Check sheet for the modelled part. Datum: model origin and axes. Units: mm. Face numbers are marked on the shaded views. A direction names the side the tool comes from. Give positions to 0.01 mm unless a question says otherwise; leave off trailing zeros. Write each loop counter-clockwise with the first axis right and the second up, starting at its lowest first coordinate (ties: lowest second). Pieces come first, ordered by that corner, then holes. Notation, with made-up numbers: M 86,16 L 103,16 A33 cw 103,46 Z; hole C 71.5,40 d2. An arc over 180 degrees is marked long. Write each question's results on one line, items separated by ' | '. Start each with the question number.
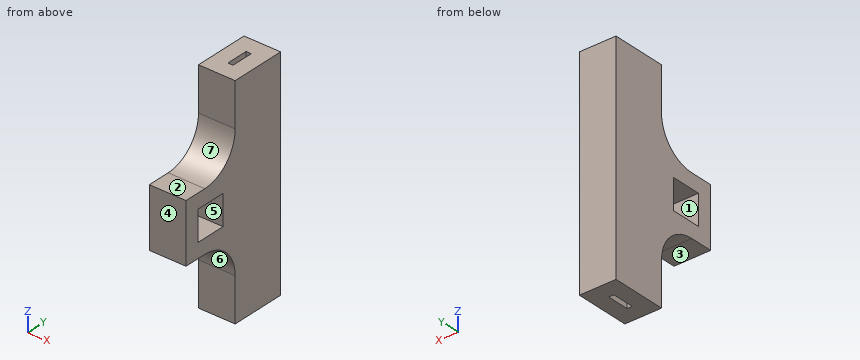
Autodesk Inventor part; units mm, degrees
ref_plane "YZ Plane" through (0, 0, 0) normal (1, 0, 0) x (0, 1, 0)
ref_plane "XZ Plane" through (0, 0, 0) normal (0, 1, 0) x (-1, 0, 0)
ref_plane "XY Plane" through (0, 0, 0) normal (0, 0, 1) x (1, 0, 0)
sketch "Sketch1" plane through (0, 0, 0) normal (1, 0, 0) x (0, 1, 0)
  line L0 (4.05, 4.05) -> (-4.05, 4.05)
  line L1 (-4.05, 4.05) -> (-4.05, -4.05)
  line L2 (-4.05, -4.05) -> (4.05, -4.05)
  line L3 (4.05, -4.05) -> (4.05, 4.05)
  line L4 (11.55, 15) -> (4.05, 15)
  line L5 (4.05, 15) -> (4.05, -15)
  line L6 (4.05, -15) -> (11.55, -15)
  line L7 (11.55, -15) -> (11.55, 15)
  line L8 (4.05, 4.05) -> (-4.05, -4.05) construction
  line L9 (4.05, -4.05) -> (-4.05, 4.05) construction
  line L10 (2.05, 2.05) -> (-2.05, 2.05)
  line L11 (-2.05, 2.05) -> (-2.05, -2.05)
  line L12 (-2.05, -2.05) -> (2.05, -2.05)
  line L13 (2.05, -2.05) -> (2.05, 2.05)
  line L14 (2.05, 2.05) -> (-2.05, -2.05) construction
  line L15 (-2.05, 2.05) -> (2.05, -2.05) construction
  point P0 (4.05, 4.05)
  point P1 (0, 0)
  point P2 (0, 0)
  point P3 (0, 0)
  dimension "d0" = 8.1
  dimension "d3" = 8.1
  dimension "d22" = 10.95
  dimension "d24" = 30
  dimension "d25" = 7.5
  dimension "d55" = 10.95
  dimension "d65" = 4.1
  dimension "d66" = 4.1
extrude "Extrusion1" add sketch "Sketch1" along normal blind 5
sketch "Sketch5" plane through (0, 4.05, 15) normal (0, 0, 1) x (1, 0, 0)
  line L0 (2.15, 5.25) -> (2.85, 5.25)
  line L1 (2.85, 5.25) -> (2.85, 2.25)
  line L2 (2.85, 2.25) -> (2.15, 2.25)
  line L3 (2.15, 2.25) -> (2.15, 5.25)
  line L4 (0, 0) -> (5, 0)
  line L5 (0, 7.5) -> (0, 0)
  point P0 (0, -4.05)
  dimension "d86" = 3
  dimension "d87" = 0.7
  dimension "d88" = 2.25
  dimension "d89" = 2.15
extrude "Extrusion4" cut sketch "Sketch5" against normal through all
fillet "Fillet3" radius 5 2 edges at (2.5, 4.05, 4.05) (2.5, 4.05, -4.05)
equation "\"d3\" = d0"
equation "\"d22\" = d55"
properties part number "fuselage_wing_interface_2" material "ABS Plastic"
Q1. Tool access check on the marked faces 1, 2, 3 and 4. Record the directions out of +Z, -Z, +X, -X, +Y, -Y that give a thin tool (end or side, any length) a straight path to the whole face; none if there is none.
Q2. Scan lines: L1, parallel to X at y = 8, z = -11.75; L2, parallel to Z at x = 1.55, y = -1.75; L3, parallel to Y at x = 2, z = -1.25. Record each from-to range of solid material in increasing order.
Q3. Section check C-C on y = 0.25. Record the boundary of the cut face in (x, z), plus the area to 3 significant figures.
Q4. Section check A-A on z = -0.5. Record the boundary of the cut face in (x, y).
Q5. Section check D-D on z = 12.75. Record the boundary of the cut face in (x, y).
Q6. Release check for a two-part mould opening along Z. For the marked faces 5, 6 and 7 record: pulls with the +Z half, pulls with the -Z half, needs draft (parallel to the pull), parting line crosses it, or undercut.
Q7. Depth check by flat-ended pin: pin 1 Ø3 at (x, z) = (0.5, -10) entering from -Y; pin 2 Ø1.5 at (y, z) = (0, -4.5) entering from +X; pin 3 Ø1.2 at (x, y) = (1.5, 0.5) entering from +Z; pin 4 Ø1.5 at (x, y) = (2, -2.5) entering from +Z. Enter the tip coordinate at first touch or a pass-through.
Q8. Section check B-B on x = 3.6. Record the boundary of the cut face in (y, z), plus the area to 3 significant figures.
Check result:
1) face 1: +X, -X | face 2: +Z, +X, -X, -Y | face 3: -Z, +X, -X, -Y | face 4: +Z, -Z, +X, -X, -Y
2) L1: 0 to 2.15, 2.85 to 5 | L2: -4.05 to -2.05, 2.05 to 4.05 | L3: -4.05 to -2.05, 2.05 to 11.55
3) outline: M 0,-4.2 L 5,-4.2 L 5,-2.05 L 0,-2.05 Z; M 0,2.05 L 5,2.05 L 5,4.2 L 0,4.2 Z | area: 21.5 mm^2
4) outline: M 0,-4.05 L 5,-4.05 L 5,-2.05 L 0,-2.05 Z; M 0,2.05 L 5,2.05 L 5,11.55 L 0,11.55 Z; hole M 2.15,6.3 L 2.85,6.3 L 2.85,9.3 L 2.15,9.3 Z
5) outline: M 0,4.05 L 5,4.05 L 5,11.55 L 0,11.55 Z; hole M 2.15,6.3 L 2.85,6.3 L 2.85,9.3 L 2.15,9.3 Z
6) face 5: undercut | face 6: pulls with the -Z half | face 7: pulls with the +Z half
7) pin 1: y = 4.02 | pin 2: x = 5 | pin 3: z = 4.49 | pin 4: z = 4.05
8) outline: M -4.05,-4.05 L -0.95,-4.05 A5 cw 4.05,-9.05 L 4.05,-15 L 11.55,-15 L 11.55,15 L 4.05,15 L 4.05,9.05 A5 cw -0.95,4.05 L -4.05,4.05 Z; hole M -2.05,-2.05 L 2.05,-2.05 L 2.05,2.05 L -2.05,2.05 Z | area: 285 mm^2
